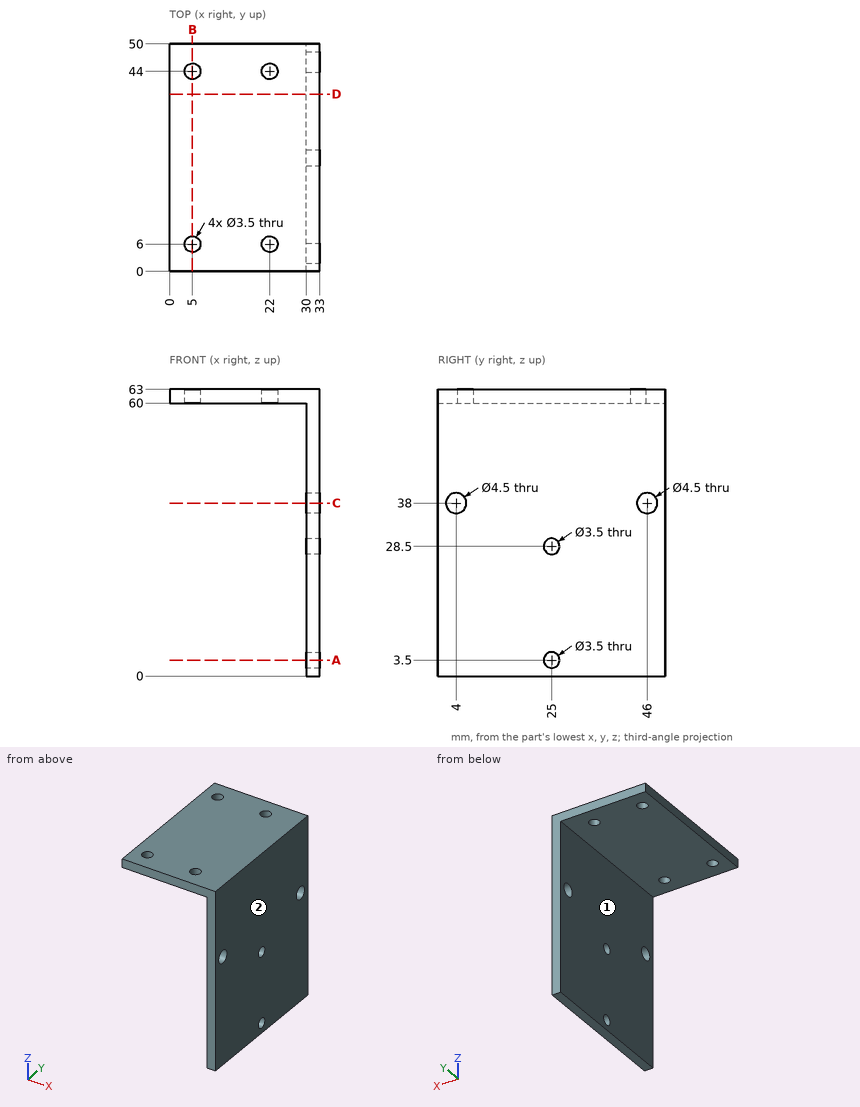
Geometry: see drawing. Coordinates: mm, zero at the bounding-box minimum. A direction names the side the tool comes from. Coordinates: 2 decimals unless noted, no trailing zeros. Loops run counter-clockwise (first coordinate to the right, second up) from the corner with the lowest first, then second, coordinate; pieces in that order, holes last. Notation, with made-up numbers: M 41,64.25 L 71,64.25 A23 ccw 71,94.25 Z; hole C -32.5,89.5 d4. An arc over 180 degrees is marked long. Answer in a Markdown table with one row per item.
1. Section B-B, the plane x = 5. Output: boundary loops of the cut face in (y, z), then the cut area to 3 significant figures.
Response:
| item | result |
|---|---|
| outline | M 0,60 L 4.25,60 L 4.25,63 L 0,63 Z; M 7.75,60 L 42.25,60 L 42.25,63 L 7.75,63 Z; M 45.75,60 L 50,60 L 50,63 L 45.75,63 Z |
| area | 129 mm2 |
2. Section C-C, the plane z = 38. Output: boundary loops of the cut face in (x, y).
Response:
| item | result |
|---|---|
| outline | M 30,0 L 33,0 L 33,1.75 L 30,1.75 Z; M 30,6.25 L 33,6.25 L 33,43.75 L 30,43.75 Z; M 30,48.25 L 33,48.25 L 33,50 L 30,50 Z |
3. First-contact query: pin 1 (3.5 mm diameter, centred on y = 4, z = 38, fed in from +X); pin 2 (5.5 mm diameter, centred on x = 5, y = 44, fed in from -Z); pin 3 (5 mm diameter, centred on y = 5, z = 32, fed in from -X). Flat tips, straight axial feed; report the tip coordinate or a pass-through.
Response:
| item | result |
|---|---|
| pin 1 | passes through |
| pin 2 | stops at z = 60 |
| pin 3 | stops at x = 30 |
4. Section A-A, the plane z = 3.5. Output: boundary loops of the cut face in (x, y), then the cut area to 4 significant figures.
Response:
| item | result |
|---|---|
| outline | M 30,0 L 33,0 L 33,23.25 L 30,23.25 Z; M 30,26.75 L 33,26.75 L 33,50 L 30,50 Z |
| area | 139.5 mm2 |
5. Material intervals for line 1 (Y direction, x = 31.35, z = 38); line 2 (X direction, y = 11, z = 32); line 3 (Z direction, x = 9.5, y = 21), sorted ascending.
Response:
| item | result |
|---|---|
| line 1 | y = 0 to 1.75, 6.25 to 43.75, 48.25 to 50 |
| line 2 | x = 30 to 33 |
| line 3 | z = 60 to 63 |
6. Section D-D, the plane y = 39. Output: boundary loops of the cut face in (x, z).
Response:
| item | result |
|---|---|
| outline | M 0,60 L 30,60 L 30,0 L 33,0 L 33,63 L 0,63 Z |
7. Reachability of the marked faces 1 and 2 from +Z, -Z, +X, -X, +Y, -Y: full face, straight path, thin tool, end or side. Return the list, or none.
Response:
| item | result |
|---|---|
| face 1 | -Z, -X, +Y, -Y |
| face 2 | +Z, -Z, +X, +Y, -Y |
